```python
from build123d import *

# Parameters (mm, degrees)
F0_W     = 35.5
F0_H     = 6
F1_DEPTH = 160
F2_W     = 35.5
F2_H     = 6
F3_DEPTH = 69.5
F5_DEPTH = 25
F6_DEPTH = 25
F8_DEPTH = 25


with BuildPart() as f1:
    # F0 (on Front) → F1 (new body)
    with BuildSketch(Plane.XZ):
        Rectangle(F0_W, F0_H)
    extrude(amount=F1_DEPTH)

    # F2 (on face) → F3 (join)
    with BuildSketch(Plane.XY.offset(3)):
        with Locations((0, -3)):
            Rectangle(F2_W, F2_H)
    extrude(amount=F3_DEPTH)

    # F4 (on face) → F5 (cut)
    with BuildSketch(Plane.XY.offset(3)):
        with BuildLine():
            Line((2.506278, -112.369976), (2.506278, -99.630027))
            ThreePointArc((2.506278, -99.630027), (0.074696, -97.000848), (-2.490338, -99.500002))
            Line((-2.490338, -99.500002), (-2.490338, -112.500002))
            ThreePointArc((-2.490338, -112.500002), (-0.055373, -114.999156), (2.506278, -112.630027))
            Line((2.506278, -112.630027), (2.506278, -112.369976))
        make_face()
    extrude(amount=-F5_DEPTH, mode=Mode.SUBTRACT)

    # F4 (on face) → F6 (cut)
    with BuildSketch(Plane.XY.offset(3)):
        with BuildLine():
            Line((2.496616, -155.369974), (2.496616, -142.630026))
            ThreePointArc((2.496616, -142.630026), (0.065035, -140.000846), (-2.5, -142.5))
            Line((-2.5, -142.5), (-2.5, -155.5))
            ThreePointArc((-2.5, -155.5), (-0.065035, -157.999154), (2.496616, -155.630026))
            Line((2.496616, -155.630026), (2.496616, -155.369974))
        make_face()
    extrude(amount=-F6_DEPTH, mode=Mode.SUBTRACT)

    # F7 (on face) → F8 (cut)
    with BuildSketch(Plane.XZ.offset(6)):
        with BuildLine():
            Line((-8.25, 52.5), (17.75, 52.5))
            Line((17.75, 52.5), (17.75, 61.5))
            Line((17.75, 61.5), (-8.25, 61.5))
            ThreePointArc((-8.25, 61.5), (-12.75, 57), (-8.25, 52.5))
        make_face()
        with BuildLine():
            Line((17.75, 21), (-8.25, 21))
            ThreePointArc((-8.25, 21), (-12.75, 16.5), (-8.25, 12))
            Line((-8.25, 12), (17.75, 12))
            Line((17.75, 12), (17.75, 21))
        make_face()
    extrude(amount=-F8_DEPTH, mode=Mode.SUBTRACT)


solid = f1.part
```
Geometry: final body of the model. Coordinates: model frame, mm. A direction names the side the tool comes from. Coordinates: 2 decimals unless noted, no trailing zeros. Order: outer loops, then holes, each group sorted by start corner. A loop starts at its lowest first (then second) coordinate and runs counter-clockwise, first axis right, second up. Notation, with made-up numbers: (85.25, 74.25) -> (94.25, 74.25) arc R26 cw to (94.25, 98.25) -> close; hole circle Ø10 at (16.5, 30). An arc over 180 degrees is marked (long way). Answer in a Markdown table with one row per item.
Item 1: Contact query for flat-ended pins moving along their axis: P1, Ø8, axis at x = -0.5, y = -98, coming from the +Z side; P2, Ø1.5, axis at x = 6, z = 35.5, coming from the -Y side. Output: stop coordinate, or through.
Return value:
| item | result |
|---|---|
| P1 | stops at z = 3 |
| P2 | stops at y = -6 |
Item 2: Section D-D on z = 57. Output: boundary loops of the cut face in (x, y), plus the area to 3 significant figures.
Return value:
| item | result |
|---|---|
| outline | (-17.75, -6) -> (-12.75, -6) -> (-12.75, 0) -> (-17.75, 0) -> close |
| area | 30.0 mm² |
Item 3: Section C-C on y = -130. Output: boundary loops of the cut face in (x, z), plus the area to 3 significant figures.
Return value:
| item | result |
|---|---|
| outline | (-17.75, -3) -> (17.75, -3) -> (17.75, 3) -> (-17.75, 3) -> close |
| area | 213 mm² |
Item 4: Access query for faces 1 (the flat face through (5, -3, 21)), 2 (the flat face through (0, 0, 34)), 3 (the flat face through (-17.75, -57, 1)), 4 (the flat face through (0, -82, 3)), 5 (the flat face through (2.506, -106, 0)). Directions: +Z, -Z, +X, -X, +Y, -Y. A direction counts if a zero-diameter tool reaches every point of the face in a straight line with its end or side. Return the directions, or none.
Return value:
| item | result |
|---|---|
| face 1 | +X, +Y, -Y |
| face 2 | +Z, -Z, +X, -X, +Y |
| face 3 | +Z, -Z, -X, +Y, -Y |
| face 4 | +Z, +X, -X, -Y |
| face 5 | +Z, -Z |
Item 5: Section B-B on x = 0. Output: boundary loops of the cut face in (y, z), plus the area to 3 significant figures.
Return value:
| item | result |
|---|---|
| outline | (-160, -3) -> (-158, -3) -> (-158, 3) -> (-160, 3) -> close; (-140, -3) -> (-115, -3) -> (-115, 3) -> (-140, 3) -> close; (-97, -3) -> (0, -3) -> (0, 12) -> (-6, 12) -> (-6, 3) -> (-97, 3) -> close; (-6, 21) -> (0, 21) -> (0, 52.5) -> (-6, 52.5) -> close; (-6, 61.5) -> (0, 61.5) -> (0, 72.5) -> (-6, 72.5) -> close |
| area | 1,050 mm² |
Item 6: Draft query along X for faces 6 (the cylindrical face through (0, -158, 0)), 7 (the flat face through (17.75, -3, 37)), 8 (the flat face through (2.497, -149, 0)), 9 (the flat face through (5, -3, 52.5)). Return one class per face: released by +X, released by -X, zero draft, split by the parting line, or undercut.
Return value:
| item | result |
|---|---|
| face 6 | undercut |
| face 7 | released by +X |
| face 8 | undercut |
| face 9 | zero draft |
Item 7: Ray query, L1, parallel to Y at x = 12.5, z = 29; L2, parallel to Z at x = -14, y = -55. Return the intervals inside material, ascending.
Return value:
| item | result |
|---|---|
| L1 | y = -6 to 0 |
| L2 | z = -3 to 3 |
Item 8: Section A-A on x = 8.5. Output: boundary loops of the cut face in (y, z).
Return value:
| item | result |
|---|---|
| outline | (-160, -3) -> (0, -3) -> (0, 12) -> (-6, 12) -> (-6, 3) -> (-160, 3) -> close; (-6, 21) -> (0, 21) -> (0, 52.5) -> (-6, 52.5) -> close; (-6, 61.5) -> (0, 61.5) -> (0, 72.5) -> (-6, 72.5) -> close |
